Autodesk Inventor part; units mm, degrees
ref_plane "YZ Plane" through (0, 0, 0) normal (1, 0, 0) x (0, 1, 0)
ref_plane "XZ Plane" through (0, 0, 0) normal (0, 1, 0) x (-1, 0, 0)
ref_plane "XY Plane" through (0, 0, 0) normal (0, 0, 1) x (1, 0, 0)
sketch "Skizze1" plane through (0, 0, 0) normal (0, 0, 1) x (1, 0, 0)
  line L0 (-86.35, 56.35) -> (86.35, 56.35)
  line L1 (86.35, 56.35) -> (86.35, -56.35)
  line L2 (86.35, -56.35) -> (-86.35, -56.35)
  line L3 (-86.35, -56.35) -> (-86.35, 56.35)
  line L4 (-86.35, 56.35) -> (86.35, -56.35) construction
  line L5 (86.35, 56.35) -> (-86.35, -56.35) construction
  point P0 (0, 0)
  dimension "d0" = 172.7
  dimension "d1" = 112.7
extrude "Extrusion1" add sketch "Skizze1" along normal blind 4
sketch "Skizze2" plane through (0, 0, 4) normal (0, 0, 1) x (1, 0, 0)
  circle A0 centre (0, 0) radius 47
  dimension "d4" = 94
extrude "Extrusion2" cut sketch "Skizze2" against normal blind 4
sketch "Skizze3" plane through (0, 0, 4) normal (0, 0, 1) x (1, 0, 0)
  circle A0 centre (-41.25, 41.25) radius 2.2
  circle A1 centre (41.25, 41.25) radius 2.2
  circle A2 centre (41.25, -41.25) radius 2.2
  circle A3 centre (-41.25, -41.25) radius 2.2
  point P0 (0, 0)
  dimension "d7" = 82.5
  dimension "d8" = 82.5
  dimension "d9" = 82.5
  dimension "d10" = 82.5
  dimension "d11" = 41.25
  dimension "d12" = 41.25
  dimension "d13" = 41.25
  dimension "d14" = 41.25
  dimension "d15" = 4.4
  dimension "d16" = 4.4
  dimension "d17" = 4.4
  dimension "d18" = 4.4
extrude "Extrusion3" cut sketch "Skizze3" against normal blind 4
sketch "Skizze4" plane through (0, 0, 4) normal (0, 0, 1) x (1, 0, 0)
  line L0 (-86.35, 56.35) -> (-46.35, 56.35)
  line L1 (-46.35, 56.35) -> (-46.35, 46.35)
  line L2 (-46.35, 46.35) -> (-86.35, 46.35)
  line L3 (-86.35, 46.35) -> (-86.35, 56.35)
  line L4 (86.35, -56.35) -> (86.35, 56.35)
  line L5 (86.35, 56.35) -> (46.35, 56.35)
  line L6 (46.35, 56.35) -> (46.35, 46.35)
  line L7 (46.35, 46.35) -> (86.35, 46.35)
  line L8 (86.35, 46.35) -> (86.35, 56.35)
  line L9 (86.35, -56.35) -> (46.35, -56.35)
  line L10 (46.35, -56.35) -> (46.35, -46.35)
  line L11 (46.35, -46.35) -> (86.35, -46.35)
  line L12 (86.35, -46.35) -> (86.35, -56.35)
  line L13 (-86.35, -56.35) -> (86.35, -56.35)
  line L14 (-86.35, -56.35) -> (-46.35, -56.35)
  line L15 (-46.35, -56.35) -> (-46.35, -46.35)
  line L16 (-46.35, -46.35) -> (-86.35, -46.35)
  line L17 (-86.35, -46.35) -> (-86.35, -56.35)
  line L18 (-86.35, 56.35) -> (-86.35, -56.35)
  point P0 (86.35, -46.35)
  point P1 (86.35, 46.35)
  dimension "d31" = 40
  dimension "d32" = 40
  dimension "d33" = 10
  dimension "d34" = 10
extrude "Extrusion4" cut sketch "Skizze4" against normal blind 10
fillet "Rundung1" radius 2 4 edges at (-46.35, 46.35, 2) (46.35, 46.35, 2) (46.35, -46.35, 2) (-46.35, -46.35, 2)
properties part number "Schutzglas_Lüfter" material "Glas"
Could you check a few things on this model? Use its own coordinates, in mm. A direction names the side the tool comes from. Round coordinates to 2 decimals unless told otherwise and drop trailing zeros. Write each loop counter-clockwise with the first axis right and the second up, starting at its lowest first coordinate (ties: lowest second). Pieces come first, ordered by that corner, then holes. Notation, with made-up numbers: M 63,37 L 84,37 A19 ccw 84,51 Z; hole C 9,-39.5 d7. An arc over 180 degrees is marked long. Answer in a Markdown table with one row per item. Add a question column.
Q1. Imagine slicing it at A-A (x = 0). Please give me the cut outline in (y, z), then the cut area to 3 significant figures.
Q2. Will these pins go through, and if not, where does the flat tip stop? pin 1 Ø5.5 at (x, y) = (41.25, 41.25) entering from -Z; pin 2 Ø2 at (y, z) = (53.5, 3) entering from -X; pin 3 Ø8 at (x, y) = (8, 41) entering from +Z; pin 4 Ø1.2 at (y, z) = (-52.5, 2.5) entering from +X.
Q3. On a 3-axis mill with a long thin cutter (end or side, diameter ignored), from which of +Z, -Z, +X, -X, +Y, -Y can I reach the whole of each face in a straight line? I mean faces 1 (the flat face through (67, -46.35, 2)), 2 (the flat face through (-46.35, 52, 2)), 3 (the flat face through (-46.35, -52, 2)). Say none if no direction works.
Q4. If I drill on line 1 (X direction, y = 0.5, z = 3.35); line 2 (Y direction, x = 41.25, z = 3.1); line 3 (Y direction, x = -43, z = 0.6), over which ranges is the centre line in solid material (lowest first)? Write a range as from..to.
Q5. Imagine slicing it at B-B (y = 0). Please give me the cut outline in (x, z), then the cut area to 3 significant figures.
Q6. If we mould it in two halves opening along X, with no side actions, what happens to faces 4 (the cylindrical face through (39.504, -42.589, 2.028)), 5 (the flat face through (46.35, -52, 2)), 6 (the flat face through (67, 46.35, 2))? For each: +X half, -X half, draft (parallel to the pull), parting line (faces both ways), or undercut.
Q7. Imagine slicing it at D-D (x = 41.25). Please give me the cut outline in (y, z), then the cut area to 3 significant figures.
Q8. Imagine slicing it at C-C (z = 2.5). Please give me the cut outline in (x, y), then the cut area to 3 significant figures.
Values:
| question | item | result |
|---|---|---|
| 1 | outline | M -56.35,0 L -47,0 L -47,4 L -56.35,4 Z; M 47,0 L 56.35,0 L 56.35,4 L 47,4 Z |
| 1 | area | 74.8 mm^2 |
| 2 | pin 1 | z = 0 |
| 2 | pin 2 | x = -46.35 |
| 2 | pin 3 | through |
| 2 | pin 4 | x = 46.35 |
| 3 | face 1 | +Z, -Z, +X, -Y |
| 3 | face 2 | +Z, -Z, -X, +Y |
| 3 | face 3 | +Z, -Z, -X, -Y |
| 4 | line 1 | -86.35..-47, 47..86.35 |
| 4 | line 2 | -56.35..-43.45, -39.05..-22.53, 22.53..39.05, 43.45..56.35 |
| 4 | line 3 | -56.35..-42.58, -39.92..-18.97, 18.97..39.92, 42.58..56.35 |
| 5 | outline | M -86.35,0 L -47,0 L -47,4 L -86.35,4 Z; M 47,0 L 86.35,0 L 86.35,4 L 47,4 Z |
| 5 | area | 315 mm^2 |
| 6 | face 4 | undercut |
| 6 | face 5 | +X half |
| 6 | face 6 | draft |
| 7 | outline | M -56.35,0 L -43.45,0 L -43.45,4 L -56.35,4 Z; M -39.05,0 L -22.53,0 L -22.53,4 L -39.05,4 Z; M 22.53,0 L 39.05,0 L 39.05,4 L 22.53,4 Z; M 43.45,0 L 56.35,0 L 56.35,4 L 43.45,4 Z |
| 7 | area | 235 mm^2 |
| 8 | outline | M -86.35,-46.35 L -48.35,-46.35 A2 cw -46.35,-48.35 L -46.35,-56.35 L 46.35,-56.35 L 46.35,-48.35 A2 cw 48.35,-46.35 L 86.35,-46.35 L 86.35,46.35 L 48.35,46.35 A2 cw 46.35,48.35 L 46.35,56.35 L -46.35,56.35 L -46.35,48.35 A2 cw -48.35,46.35 L -86.35,46.35 Z; hole C 0,0 d94; hole C -41.25,-41.25 d4.4; hole C -41.25,41.25 d4.4; hole C 41.25,-41.25 d4.4; hole C 41.25,41.25 d4.4 |
| 8 | area | 10,900 mm^2 |
